The listing builds one solid part. Answer for the finished solid, in the listing's coordinates (mm). Face numbers are marked on the shaded views. A direction names the side the tool comes from. Give positions to 0.01 mm unless a question says otherwise; leave off trailing zeros. Write each loop counter-clockwise with the first axis right and the second up, starting at its lowest first coordinate (ties: lowest second). Pieces come first, ordered by that corner, then holes. Notation, with made-up numbers: M 76,-40 L 123,-40 A33 ccw 123,-8 Z; hole C 21,-22.5 d3. An arc over 180 degrees is marked long. Answer as a JSON object with one key per item and string values.
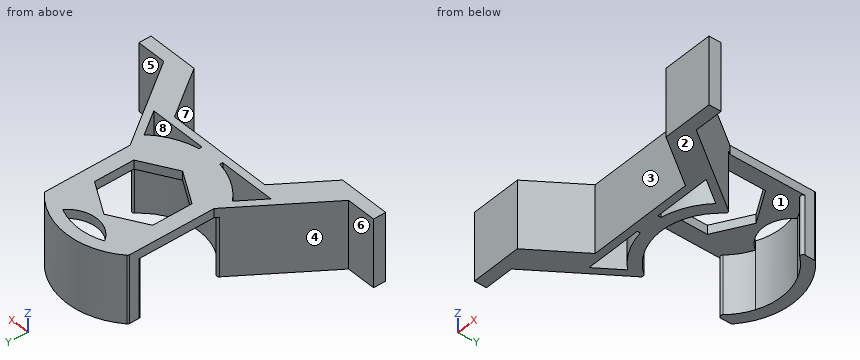
```python
from build123d import *

# Parameters (mm, degrees)
BOSS_EXTRU_1_DEPTH      = 28
ESQUISSE2_R             = 24.75
ENL_V_MAT_EXTRU_1_DEPTH = 24.3
ENL_V_MAT_EXTRU_6_DEPTH = 29
CONG_1_R                = 1


with BuildPart() as part:
    # Esquisse1 → Boss.-Extru.1 (new body)
    with BuildSketch(Plane.XY):
        with BuildLine():
            Line((-56.5, 0), (-56.5, 5))
            Line((-56.5, 5), (-44.5, 5))
            Line((-44.5, 5), (-20.262248583, 39.527154166))
            Line((-20.262248583, 39.527154166), (-20.262248583, 74.740412365))
            ThreePointArc((-20.262248583, 74.740412365), (0, 82.8), (20.262248583, 74.740412365))
            Line((20.262248583, 74.740412365), (20.262248583, 39.527154166))
            Line((20.262248583, 39.527154166), (44.5, 5))
            Line((44.5, 5), (56.5, 5))
            Line((56.5, 5), (56.5, 0))
            Line((56.5, 0), (35.791970863, 0))
            Line((35.791970863, 0), (21.7521509, 20))
            Line((21.7521509, 20), (-21.7521509, 20))
            Line((-21.7521509, 20), (-35.791970863, 0))
            Line((-35.791970863, 0), (-56.5, 0))
        make_face()
    extrude(amount=BOSS_EXTRU_1_DEPTH)

    # Esquisse2 → Enlèv. mat.-Extru.1 (cut)
    with BuildSketch(Plane.XY):
        with Locations((0, 53.3)):
            Circle(ESQUISSE2_R)
    extrude(amount=ENL_V_MAT_EXTRU_1_DEPTH, mode=Mode.SUBTRACT)

    # Esquisse5 → Enlèv. mat.-Extru.6 (cut, through all)
    with BuildSketch(Plane.XY.offset(28)):
        Polygon((0, 67.565807537), (-14, 59.482903769), (-14, 43.317096231), (0, 35.234192463), (14, 43.317096231), (14, 59.482903769), align=None)
        with BuildLine():
            Line((-21.274554731, 32.863676431), (-28.198766795, 23))
            Line((-28.198766795, 23), (-5, 23))
            Line((-5, 23), (-5, 24.22681648))
            ThreePointArc((-5, 24.22681648), (-13.828842831, 27.242120079), (-21.274554731, 32.863676431))
        make_face()
        with BuildLine():
            Line((21.274554731, 32.863676431), (28.198766795, 23))
            Line((28.198766795, 23), (5, 23))
            Line((5, 23), (5, 24.22681648))
            ThreePointArc((5, 24.22681648), (13.828842831, 27.242120079), (21.274554731, 32.863676431))
        make_face()
        with BuildLine():
            ThreePointArc((-10.099699908, 75.895542962), (0, 70.565807537), (10.099699908, 75.895542962))
            ThreePointArc((10.099699908, 75.895542962), (0, 78.05), (-10.099699908, 75.895542962))
        make_face()
    extrude(amount=-ENL_V_MAT_EXTRU_6_DEPTH, mode=Mode.SUBTRACT)

    # Congé1
    cong_1_edges = [part.edges().sort_by_distance(p)[0] for p in [
        (-20.262248583, 74.740412365, 14),
        (20.262248583, 74.740412365, 14),
        (20.415715975, 39.308536844, 12.15),
        (20.262248583, 67.512803466, 12.15),
        (-20.262248583, 67.512803466, 12.15),
        (-20.415715975, 39.308536844, 12.15),
    ]]
    fillet(cong_1_edges, radius=CONG_1_R)


solid = part.part
```
1. Flat-ended cylindrical pins translate along their axes: pin 1 (1.8 mm diameter, centred on y = 51.5, z = 26, fed in from -X); pin 2 (11.5 mm diameter, centred on x = 20, z = 18.5, fed in from +Y); pin 3 (1 mm diameter, centred on y = 23.5, z = 8.5, fed in from +X). Find the tip coordinate at first contact, or state that the pin passes through.
Verdict:
{"pin 1": "stops at x = -20.26", "pin 2": "stops at y = 79.13", "pin 3": "stops at x = 31.86"}
2. The mould has two halves that part along X. Classify the marked faces 1, 2, 3 and 4: released by +X, released by -X, zero draft, split by the parting line, or undercut.
Verdict:
{"face 1": "undercut", "face 2": "zero draft", "face 3": "undercut", "face 4": "released by -X"}
3. A cutting plane is placed at C-C, the plane y = 18. Give the vertices of the cut face in (x, z).
Verdict:
{"outline": "M -35.37,0 L -23.16,0 L -23.16,28 L -35.37,28 Z; M 23.16,0 L 35.37,0 L 35.37,28 L 23.16,28 Z"}
4. Consider line 1 along Y through (x, z) = (-10, 23); line 2 along Y through (x, z) = (7, 5.5); line 3 along Y through (x, z) = (45, 3.5). Determine where each line is inside the solid, lowest interval first.
Verdict:
{"line 1": "y = 20 to 23, 25.55 to 30.66, 75.94 to 81.05", "line 2": "y = 20 to 23, 24.64 to 29.56, 77.04 to 81.96", "line 3": "y = 0 to 5"}
5. A cutting plane is placed at A-A, the plane z = 12.5. Count the separate pieces of the cut face and the enclosed holes in it, plus the area to 3 significant figures.
Verdict:
{"separate pieces": "2", "enclosed holes": "2", "area": "1,330 mm2"}
6. For the marked faces 5, 6, 7 and 8, determine the directions among +Z, -Z, +X, -X, +Y, -Y from which every point of the face is accessible in a straight line to the end or side of a thin tool.
Verdict:
{"face 5": "+Z, -Z, +X, +Y", "face 6": "+Z, -Z, -X, +Y", "face 7": "+Z, -Z, -Y", "face 8": "+Z, -Z"}
7. A cutting plane is placed at D-D, the plane x = -24. Give the vertices of the cut face in (y, z).
Verdict:
{"outline": "M 16.8,0 L 23,0 L 23,28 L 16.8,28 Z; M 28.98,0 L 34.2,0 L 34.2,28 L 28.98,28 Z"}
